Here's the drawing with two shaded views (mm, measured from the low corner). I have some questions. Round coordinates to 2 decimals unless told otherwise and drop trailing zeros. Write each loop counter-clockwise with the first axis right and the second up, starting at its lowest first coordinate (ties: lowest second). Pieces come first, ordered by that corner, then holes.
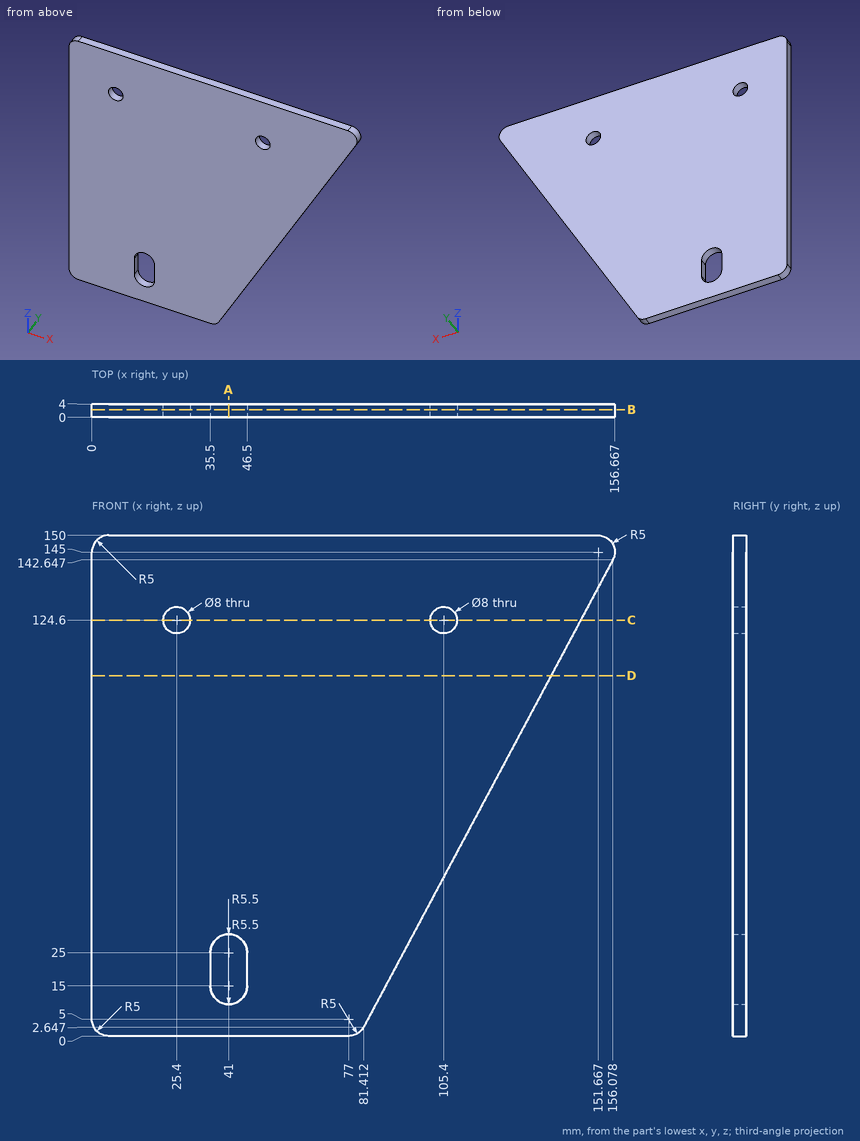
Q1. I'm going to push flat-ended pins straight in: pin 1 Ø5 at (x, z) = (25.4, 124.6) entering from -Y; pin 2 Ø1.2 at (y, z) = (1, 18) entering from +X; pin 3 Ø2 at (y, z) = (3, 94) entering from -X. Where does each tip first touch, or does it pass through?
Q2. Imagine slicing it at D-D, the plane z = 108. Write out the boundary of the cut face in (x, y).
Q3. Imagine slicing it at C-C, the plane z = 124.6. Write out the boundary of the cut face in (x, y), then the cut area to 3 significant figures.
Q4. Imagine slicing it at B-B, the plane y = 2.35. Write out the boundary of the cut face in (x, z).
Q5. If I drill on L1, parallel to Z at x = 40.5, y = 1.1; L2, parallel to Z at x = 25.4, y = 3; L3, parallel to X at y = 1.6, z = 124.6 (1 decimal), over which ranges is the centre line in solid material (lowest first)?
Q6. Imagine slicing it at A-A, the plane x = 41. Write out the boundary of the cut face in (y, z), then the cut area to 3 significant figures.
Results found:
1. pin 1: passes through
1. pin 2: stops at x = 89.92
1. pin 3: stops at x = 0
2. outline: (0, 0) - (137.6, 0) - (137.6, 4) - (0, 4) - close
3. outline: (0, 0) - (21.4, 0) - (21.4, 4) - (0, 4) - close; (29.4, 0) - (101.4, 0) - (101.4, 4) - (29.4, 4) - close; (109.4, 0) - (146.45, 0) - (146.45, 4) - (109.4, 4) - close
3. area: 522 mm2
4. outline: (0, 5) arc R5 ccw to (5, 0) - (77, 0) arc R5 ccw to (81.41, 2.65) - (156.08, 142.65) arc R5 ccw to (151.67, 150) - (5, 150) arc R5 ccw to (0, 145) - close; hole circle Ø8 at (25.4, 124.6); hole (35.5, 15) arc R5.5 ccw to (46.5, 15) - (46.5, 25) arc R5.5 ccw to (35.5, 25) - close; hole circle Ø8 at (105.4, 124.6)
5. L1: z = 0 to 9.52, 30.48 to 150
5. L2: z = 0 to 120.6, 128.6 to 150
5. L3: x = 0 to 21.4, 29.4 to 101.4, 109.4 to 146.5
6. outline: (0, 0) - (4, 0) - (4, 9.5) - (0, 9.5) - close; (0, 30.5) - (4, 30.5) - (4, 150) - (0, 150) - close
6. area: 516 mm2
